Verification items for the finished model (mm, model axes). Face numbers are marked on the shaded views. A direction names the side the tool comes from. Round coordinates to 2 decimals unless told otherwise and drop trailing zeros. Loops run counter-clockwise (first coordinate to the right, second up) from the corner with the lowest first, then second, coordinate; pieces in that order, holes last. Notation, with made-up numbers: (-3, 35) -> (13, 35) arc R14 ccw to (13, 48) -> close; hole circle Ø5 at (67.25, -1). An arc over 180 degrees is marked (long way). Write item = value, one per line.
```python
from build123d import *

# Parameters (mm, degrees)
F0_W      = 42.037
F0_H      = 31.8008
F1_DEPTH  = 5.08
F2_W      = 40.005
F2_H      = 29.7688
F3_DEPTH  = 3.81
F4_W      = 2.54
F4_H      = 3.556
F5_DEPTH  = 5.08
F6_W      = 2.54
F6_H      = 3.556
F7_DEPTH  = 2.54
F8_W      = 2.54
F8_H      = 3.556
F9_DEPTH  = 5.08
F10_W     = 2.54
F10_H     = 3.556
F11_DEPTH = 2.54
F12_W     = 2.54
F12_H     = 3.556
F13_DEPTH = 5.08
F14_W     = 2.54
F14_H     = 3.556
F15_DEPTH = 2.54
F16_W     = 2.54
F16_H     = 3.556
F17_DEPTH = 5.08
F18_W     = 2.54
F18_H     = 3.556
F19_DEPTH = 2.54
F20_W     = 11.557
F20_H     = 3.81
F21_DEPTH = 1.016
F22_W     = 6.4008
F22_H     = 1.27
F23_DEPTH = 6.35
F24_W     = 6.4008
F24_H     = 1.27
F25_DEPTH = 6.35
F26_R     = 1.29794
F27_DEPTH = 1.271
F28_R     = 1.29794
F29_DEPTH = 1.27


with BuildPart() as f1:
    # F0 (on Top) → F1 (new body)
    with BuildSketch(Plane.XY):
        Rectangle(F0_W, F0_H)
    extrude(amount=F1_DEPTH)

    # F2 (on face) → F3 (cut)
    with BuildSketch(Plane.XY.offset(5.08)):
        Rectangle(F2_W, F2_H)
    extrude(amount=-F3_DEPTH, mode=Mode.SUBTRACT)

    # F4 (on face) → F5 (join)
    with BuildSketch(Plane(origin=(0, -14.8844, 0), x_dir=(-1, 0, 0), z_dir=(0, 1, 0))):
        with Locations((-18.7325, 3.048)):
            Rectangle(F4_W, F4_H)
    extrude(amount=F5_DEPTH)

    # F6 (on face) → F7 (join)
    with BuildSketch(Plane.YZ.offset(-17.4625)):
        with Locations((13.6144, 3.048)):
            Rectangle(F6_W, F6_H)
    extrude(amount=F7_DEPTH)

    # F8 (on face) → F9 (join)
    with BuildSketch(Plane.YZ.offset(-20.0025)):
        with Locations((-13.6144, 3.048)):
            Rectangle(F8_W, F8_H)
    extrude(amount=F9_DEPTH)

    # F10 (on face) → F11 (join)
    with BuildSketch(Plane.XZ.offset(-12.3444)):
        with Locations((18.7325, 3.048)):
            Rectangle(F10_W, F10_H)
    extrude(amount=F11_DEPTH)

    # F12 (on face) → F13 (join)
    with BuildSketch(Plane.XZ.offset(-14.8844)):
        with Locations((-18.7325, 3.048)):
            Rectangle(F12_W, F12_H)
    extrude(amount=F13_DEPTH)

    # F14 (on face) → F15 (join)
    with BuildSketch(Plane(origin=(17.4625, 0, 0), x_dir=(0, -1, 0), z_dir=(-1, 0, 0))):
        with Locations((13.6144, 3.048)):
            Rectangle(F14_W, F14_H)
    extrude(amount=F15_DEPTH)

    # F16 (on face) → F17 (join)
    with BuildSketch(Plane(origin=(20.0025, 0, 0), x_dir=(0, -1, 0), z_dir=(-1, 0, 0))):
        with Locations((-13.6144, 3.048)):
            Rectangle(F16_W, F16_H)
    extrude(amount=F17_DEPTH)

    # F18 (on face) → F19 (join)
    with BuildSketch(Plane(origin=(0, -12.3444, 0), x_dir=(-1, 0, 0), z_dir=(0, 1, 0))):
        with Locations((18.7325, 3.048)):
            Rectangle(F18_W, F18_H)
    extrude(amount=F19_DEPTH)

    # F20 (on face) → F21 (cut, through all)
    with BuildSketch(Plane.XZ.offset(15.9004)):
        with Locations((0, 3.175)):
            Rectangle(F20_W, F20_H)
    extrude(amount=-F21_DEPTH, mode=Mode.SUBTRACT)

    # F22 (on face) → F23 (join)
    with BuildSketch(Plane.YZ.offset(21.0185)):
        with Locations((0, 0.635)):
            Rectangle(F22_W, F22_H)
    extrude(amount=F23_DEPTH)

    # F24 (on face) → F25 (join)
    with BuildSketch(Plane(origin=(-21.0185, 0, 0), x_dir=(0, -1, 0), z_dir=(-1, 0, 0))):
        with Locations((0, 0.635)):
            Rectangle(F24_W, F24_H)
    extrude(amount=F25_DEPTH)

    # F26 (on face) → F27 (cut, through all)
    with BuildSketch(Plane.XY.offset(1.27)):
        with Locations((24.1935, 0)):
            Circle(F26_R)
    extrude(amount=-F27_DEPTH, mode=Mode.SUBTRACT)

    # F28 (on face) → F29 (cut, through all)
    with BuildSketch(Plane.XY.offset(1.27)):
        with Locations((-24.1935, 0)):
            Circle(F28_R)
    extrude(amount=-F29_DEPTH, mode=Mode.SUBTRACT)


solid = f1.part
```
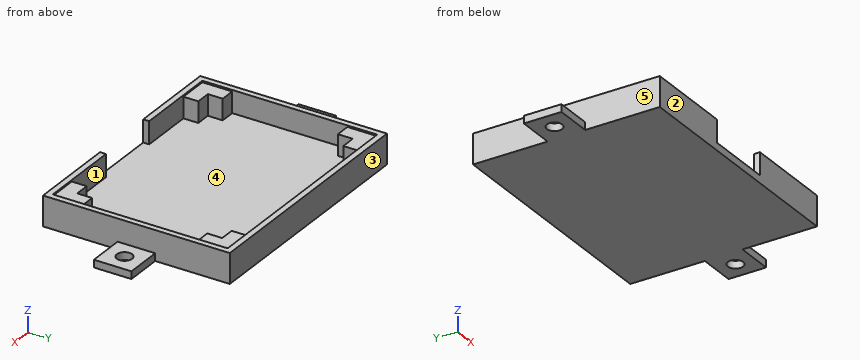
(1) Sectioned sample at A-A, the plane y = 0. Record the cut outline in (x, z).
Filled sheet:
outline = (-27.37, 0) -> (-25.49, 0) -> (-25.49, 1.27) -> (-27.37, 1.27) -> close; (-22.9, 0) -> (22.9, 0) -> (22.9, 1.27) -> (21.02, 1.27) -> (21.02, 5.08) -> (20, 5.08) -> (20, 1.27) -> (-20, 1.27) -> (-20, 5.08) -> (-21.02, 5.08) -> (-21.02, 1.27) -> (-22.9, 1.27) -> close; (25.49, 0) -> (27.37, 0) -> (27.37, 1.27) -> (25.49, 1.27) -> close
(2) Set-up check for the marked faces 1 and 2: record each of +Z, -Z, +X, -X, +Y, -Y from which the full face is reachable in a straight line by a thin tool's end or side.
Filled sheet:
face_1 = +Z
face_2 = +Z, -Z, +X, -X, -Y
(3) Sectioned sample at C-C, the plane z = 2.4. Record the cut outline in (x, y).
Filled sheet:
outline = (-21.02, -15.9) -> (-5.78, -15.9) -> (-5.78, -14.88) -> (-14.92, -14.88) -> (-14.92, -12.34) -> (-17.46, -12.34) -> (-17.46, -9.8) -> (-20, -9.8) -> (-20, 9.8) -> (-17.46, 9.8) -> (-17.46, 12.34) -> (-14.92, 12.34) -> (-14.92, 14.88) -> (14.92, 14.88) -> (14.92, 12.34) -> (17.46, 12.34) -> (17.46, 9.8) -> (20, 9.8) -> (20, -9.8) -> (17.46, -9.8) -> (17.46, -12.34) -> (14.92, -12.34) -> (14.92, -14.88) -> (5.78, -14.88) -> (5.78, -15.9) -> (21.02, -15.9) -> (21.02, 15.9) -> (-21.02, 15.9) -> close
(4) Material ranges on probe 1 along X at (y, z) = (0, 1.85); probe 2 along Y at (x, z) = (-12.5, 3.15); probe 3 along X at (y, z) = (13, 3.4), recorded low to high. Write a range as from..to.
Filled sheet:
probe_1 = -21.02..-20, 20..21.02
probe_2 = -15.9..-14.88, 14.88..15.9
probe_3 = -21.02..-14.92, 14.92..21.02
(5) Sectioned sample at D-D, the plane x = -2.5. Record the cut outline in (y, z), and give its area (3 significant figures).
Filled sheet:
outline = (-15.9, 0) -> (15.9, 0) -> (15.9, 5.08) -> (14.88, 5.08) -> (14.88, 1.27) -> (-15.9, 1.27) -> close
area = 44.3 mm2
(6) Draft check along Y on the marked faces 3, 4 and 5. Enter one of: released by +Y, released by -Y, zero draft, split by the parting line, or undercut.
Filled sheet:
face_3 = released by +Y
face_4 = undercut
face_5 = zero draft
(7) Sectioned sample at B-B, the plane x = 8. Record the cut outline in (y, z), and give its area (3 significant figures).
Filled sheet:
outline = (-15.9, 0) -> (15.9, 0) -> (15.9, 5.08) -> (14.88, 5.08) -> (14.88, 1.27) -> (-14.88, 1.27) -> (-14.88, 5.08) -> (-15.9, 5.08) -> close
area = 48.1 mm2
(8) Go/stop test with flat-tipped pins: pin 1 Ø1.5 at (x, y) = (-18.5, 13) entering from +Z; pin 2 Ø2 at (x, z) = (2.5, 4) entering from -Y; pin 3 Ø2 at (y, z) = (11, 3.5) entering from -X. Record where each tip stops, or that it passes through.
Filled sheet:
pin_1 = 4.83
pin_2 = 14.88
pin_3 = -21.02
